```python
from build123d import *

# Parameters (mm, degrees)
BOSS_EXTRUDE1_DEPTH = 400
FILLET1_R           = 12.7
BOSS_EXTRUDE3_DEPTH = 110
FILLET2_R           = 12.7


with BuildPart() as part:
    # Sketch1 → Boss-Extrude1 (new body)
    with BuildSketch(Plane(origin=(0, 0, 0), x_dir=(1, 0, 0), z_dir=(0, 1, 0))):
        with BuildLine():
            Line((25.4, 0), (426.6, 0))
            ThreePointArc((426.6, 0), (444.560512242, 7.439487758), (452, 25.4))
            Line((452, 25.4), (452, 214.6))
            ThreePointArc((452, 214.6), (444.560512242, 232.560512242), (426.6, 240))
            Line((426.6, 240), (25.4, 240))
            ThreePointArc((25.4, 240), (7.439487758, 232.560512242), (0, 214.6))
            Line((0, 214.6), (0, 25.4))
            ThreePointArc((0, 25.4), (7.439487758, 7.439487758), (25.4, 0))
        make_face()
    extrude(amount=BOSS_EXTRUDE1_DEPTH)

    # Fillet1
    fillet1_edges = [part.edges().sort_by_distance(p)[0] for p in [
        (226, 0, 0),
        (7.439487758, 0, -7.439487758),
        (0, 0, -120),
        (7.439487758, 0, -232.560512242),
        (7.439487758, 400, -7.439487758),
        (226, 400, 0),
        (444.560512242, 400, -7.439487758),
        (452, 400, -120),
        (444.560512242, 400, -232.560512242),
        (226, 400, -240),
        (7.439487758, 400, -232.560512242),
        (226, 0, -240),
        (0, 400, -120),
        (444.560512242, 0, -232.560512242),
        (452, 0, -120),
        (444.560512242, 0, -7.439487758),
    ]]
    fillet(fillet1_edges, radius=FILLET1_R)

    # Sketch2 → Boss-Extrude3 (add)
    with BuildSketch(Plane(origin=(0, 400, 0), x_dir=(1, 0, 0), z_dir=(0, 1, 0))):
        with BuildLine():
            Line((50.8, 25.4), (401.2, 25.4))
            ThreePointArc((401.2, 25.4), (419.160512242, 32.839487758), (426.6, 50.8))
            Line((426.6, 50.8), (426.6, 189.2))
            ThreePointArc((426.6, 189.2), (419.160512242, 207.160512242), (401.2, 214.6))
            Line((401.2, 214.6), (50.8, 214.6))
            ThreePointArc((50.8, 214.6), (32.839487758, 207.160512242), (25.4, 189.2))
            Line((25.4, 189.2), (25.4, 50.8))
            ThreePointArc((25.4, 50.8), (32.839487758, 32.839487758), (50.8, 25.4))
        make_face()
    extrude(amount=BOSS_EXTRUDE3_DEPTH)

    # Fillet2
    fillet2_edges = [part.edges().sort_by_distance(p)[0] for p in [
        (419.160512242, 510, -207.160512242),
        (226, 510, -214.6),
        (32.839487758, 510, -207.160512242),
        (25.4, 510, -120),
        (32.839487758, 510, -32.839487758),
        (226, 510, -25.4),
        (419.160512242, 510, -32.839487758),
        (426.6, 510, -120),
    ]]
    fillet(fillet2_edges, radius=FILLET2_R)


solid = part.part
```
Geometry check sheet. Reference: the model listing, model coordinates, mm. A direction names the side the tool comes from. Coordinates: 2 decimals unless noted, no trailing zeros. Order: outer loops, then holes, each group sorted by start corner. A loop starts at its lowest first (then second) coordinate and runs counter-clockwise, first axis right, second up.
Item 1: Tool access check on faces 1 (the flat face through (228, 448, -214.6)), 2 (the cylindrical face through (32.64, 447.97, -33.04)), 3 (the flat face through (224, 448, -25.4)), 4 (the flat face through (426.6, 448, -119)), 5 (the flat face through (209, 400, -25)). Record the directions out of +Z, -Z, +X, -X, +Y, -Y that give a thin tool (end or side, any length) a straight path to the whole face; none if there is none.
Item 2: Depth check by flat-ended pin: pin 1 (1 mm diameter, centred on y = 457.5, z = -80, fed in from -X); pin 2 (1 mm diameter, centred on y = 442, z = -138.5, fed in from +X); pin 3 (1 mm diameter, centred on x = 54.5, y = 458, fed in from +Z). Enter the tip coordinate at first touch or a pass-through.
Item 3: Section check A-A (y = 413). Enter the section's corners in (x, z), plus the area to 3 significant figures.
Item 4: Section check B-B (z = -67). Enter the section's corners in (x, y), plus the area to 3 significant figures.
Item 5: Scan lines: line 1 along Z through (x, y) = (193.5, 415); line 2 along Y through (x, z) = (368, -219.5); line 3 along Z through (x, y) = (429, 357). Record each from-to range of solid material in increasing order.
Item 6: Section check C-C (x = 220). Enter the section's corners in (y, z), plus the area to 3 significant figures.
Check sheet entries:
1. face 1: -Z, +X, -X, +Y
1. face 2: +Z, -X, +Y
1. face 3: +Z, +X, -X, +Y
1. face 4: +Z, -Z, +X, +Y
1. face 5: +Y
2. pin 1: stops at x = 25.4
2. pin 2: stops at x = 426.6
2. pin 3: stops at z = -25.4
3. outline: (25.4, -189.2) arc R25.4 ccw to (50.8, -214.6) - (401.2, -214.6) arc R25.4 ccw to (426.6, -189.2) - (426.6, -50.8) arc R25.4 ccw to (401.2, -25.4) - (50.8, -25.4) arc R25.4 ccw to (25.4, -50.8) - close
3. area: 75,400 mm2
4. outline: (0, 12.7) arc R12.7 ccw to (12.7, 0) - (439.3, 0) arc R12.7 ccw to (452, 12.7) - (452, 387.3) arc R12.7 ccw to (439.3, 400) - (426.6, 400) - (426.6, 497.3) arc R12.7 ccw to (413.9, 510) - (38.1, 510) arc R12.7 ccw to (25.4, 497.3) - (25.4, 400) - (12.7, 400) arc R12.7 ccw to (0, 387.3) - close
4. area: 225,000 mm2
5. line 1: z = -214.6 to -25.4
5. line 2: y = 0 to 400
5. line 3: z = -239.89 to -0.11
6. outline: (0, -227.3) arc R12.7 ccw to (12.7, -240) - (387.3, -240) arc R12.7 ccw to (400, -227.3) - (400, -214.6) - (497.3, -214.6) arc R12.7 ccw to (510, -201.9) - (510, -38.1) arc R12.7 ccw to (497.3, -25.4) - (400, -25.4) - (400, -12.7) arc R12.7 ccw to (387.3, 0) - (12.7, 0) arc R12.7 ccw to (0, -12.7) - close
6. area: 117,000 mm2
